Read the model definition and answer for the solid it produces. Units are mm, in the model's axes. Give positions to 0.01 mm unless a question says otherwise; leave off trailing zeros. Loops run counter-clockwise (first coordinate to the right, second up) from the corner with the lowest first, then second, coordinate; pieces in that order, holes last. Notation, with made-up numbers: (-23, 21.5) - (7, 21.5) arc R19 ccw to (7, 50.5) - close; hole circle Ø4 at (29.5, 15). An arc over 180 degrees is marked (long way). Use a Markdown table: item, result. Add a question column.
Item 1: A cutting plane is placed at B-B (y = 156.5). Determine the outline of the cut face in (x, z).
Item 2: A cutting plane is placed at A-A (x = -61). Determine the outline of the cut face in (y, z).
Item 3: Each of these flat-tipped pins is pushed along its axis until it touches: P1, Ø8, axis at x = -175, z = 13, coming from the -Y side; P2, Ø4, axis at y = -0.5, z = 42, coming from the -X side; P3, Ø10, axis at y = 182.5, z = 33.5, coming from the +X side. Where does it stop, or does it pass through?
Item 4: A cutting plane is placed at D-D (z = 12.5). Determine the outline of the cut face in (x, y), plus the area to 3 significant figures.
Item 5: Consider probe 1 along X at (y, z) = (-75.5, 23.5); probe 2 along Y at (x, z) = (-23.5, 40); probe 3 along X at (y, z) = (150, 26). Determine where each line is inside the solid, lowest interval first. Write a range as [from, to].
Item 6: A cutting plane is placed at C-C (z = 50). Determine the outline of the cut face in (x, y).
from build123d import *
from OCP.BRepAlgoAPI import BRepAlgoAPI_Cut
from OCP.TopTools import TopTools_ListOfShape

# Parameters (mm, degrees)
SKETCH1_W           = 500
SKETCH1_H           = 500
BOSS_EXTRUDE1_DEPTH = 60
FILLET3_R           = 50
FILLET4_R           = 50
FILLET6_START       = -234
FILLET6_DEPTH       = 502
FILLET6_2_DEPTH     = 492


with BuildPart() as part:
    # Sketch1 → Boss-Extrude1 (new body)
    with BuildSketch(Plane.XY):
        with Locations((11.616161616, 16.666666667)):
            Rectangle(SKETCH1_W, SKETCH1_H)
    extrude(amount=BOSS_EXTRUDE1_DEPTH)

    # Fillet3
    fillet3_edges = [part.edges().sort_by_distance(p)[0] for p in [
        (11.616161616, -233.333333333, 60),
        (261.616161616, 16.666666667, 60),
        (11.616161616, 266.666666667, 60),
        (-238.383838384, 16.666666667, 60),
    ]]
    fillet(fillet3_edges, radius=FILLET3_R)

    # Fillet4
    # the kernel refuses this fillet: 50 mm, written as the material it takes off along each edge
    with BuildSketch(Plane(origin=(-238.383838384, 341.666666667, 0), x_dir=(0, 0, 1), z_dir=(0, -1, 0)), Plane(origin=(336.616161616, 266.666666667, 0), x_dir=(0, 0, 1), z_dir=(-1, 0, 0))) as fillet4_piece_1:
        with BuildLine():
            CenterArc((50, -30), FILLET4_R, 143.130102354, 36.869897646)
            Line((0, -30), (-1, -30))
            Line((-1, -30), (-1, 0))
            Line((-1, 0), (0, 1))
            ThreePointArc((0, 1), (5, 1), (9.2, 0.6))
            Line((9.2, 0.6), (10, 0))
        make_face()
    extrude(amount=650, mode=Mode.SUBTRACT)
    with BuildSketch(Plane(origin=(-313.383838384, -233.333333333, 0), x_dir=(0, 1, 0), z_dir=(1, 0, 0)), Plane(origin=(261.616161616, -308.333333333, 0), x_dir=(-1, 0, 0), z_dir=(0, 1, 0))) as fillet4_piece_2:
        with BuildLine():
            CenterArc((30, 50), FILLET4_R, 233.130102354, 36.869897646)
            Line((0, 10), (-0.6, 9.2))
            ThreePointArc((-0.6, 9.2), (-1, 5), (-1, 0))
            Line((-1, 0), (0, -1))
            Line((0, -1), (30, -1))
            Line((30, -1), (30, 0))
        make_face()
    extrude(amount=650, mode=Mode.SUBTRACT)


with BuildPart() as fillet6_tool:
    # Fillet6: read off the stored shape, not the designer's step
    # Fillet6 outline → Fillet6 (new body)
    with BuildSketch(Plane(origin=(0, 0, 0), x_dir=(1, 0, 0), z_dir=(0, 1, 0)).offset(FILLET6_START)):
        with BuildLine():
            ThreePointArc((261.616161616, -10), (247.427549917, -2.565835097), (231.616161616, 0))
            ThreePointArc((231.616161616, 0), (253.976841391, -13.819660113), (251.616161616, -40))
            ThreePointArc((251.616161616, -40), (259.050326518, -25.811388301), (261.616161616, -10))
        make_face()
        with BuildLine():
            ThreePointArc((-228.383838384, -40), (-230.744518159, -13.819660113), (-208.383838384, 0))
            ThreePointArc((-208.383838384, 0), (-224.195226685, -2.565835097), (-238.383838384, -10))
            ThreePointArc((-238.383838384, -10), (-235.818003286, -25.811388301), (-228.383838384, -40))
        make_face()
    extrude(amount=FILLET6_DEPTH)


with BuildPart() as part_1:
    add(part.part)

    # Fillet6: cut by fillet6_tool, with a tolerance
    fillet6_stock = TopTools_ListOfShape()
    fillet6_stock.Append(part_1.part.wrapped)
    fillet6_tools = TopTools_ListOfShape()
    fillet6_tools.Append(fillet6_tool.part.wrapped)
    fillet6_cut = BRepAlgoAPI_Cut()
    fillet6_cut.SetArguments(fillet6_stock)
    fillet6_cut.SetTools(fillet6_tools)
    fillet6_cut.SetFuzzyValue(0.00001)
    fillet6_cut.Build()
    add(Compound.cast(fillet6_cut.Shape()).solids(), mode=Mode.REPLACE)


with BuildPart() as fillet6_2_tool:
    # Fillet6 2 outline → Fillet6 2 (new body)
    with BuildSketch(Plane.YZ.offset(FILLET6_START)):
        with BuildLine():
            ThreePointArc((-233.333333333, 10), (-219.144721634, 2.565835097), (-203.333333333, 0))
            ThreePointArc((-203.333333333, 0), (-225.694013108, 13.819660113), (-223.333333333, 40))
            ThreePointArc((-223.333333333, 40), (-230.767498236, 25.811388301), (-233.333333333, 10))
        make_face()
        with BuildLine():
            ThreePointArc((256.666666667, 40), (259.027346442, 13.819660113), (236.666666667, 0))
            ThreePointArc((236.666666667, 0), (252.478054612, 2.565834979), (266.666666667, 10))
            ThreePointArc((266.666666667, 10), (264.100831569, 25.811388301), (256.666666667, 40))
        make_face()
    extrude(amount=FILLET6_2_DEPTH)


with BuildPart() as part_2:
    add(part_1.part)

    # Fillet6 2: cut by fillet6_2_tool, with a tolerance
    fillet6_2_stock = TopTools_ListOfShape()
    fillet6_2_stock.Append(part_2.part.wrapped)
    fillet6_2_tools = TopTools_ListOfShape()
    fillet6_2_tools.Append(fillet6_2_tool.part.wrapped)
    fillet6_2_cut = BRepAlgoAPI_Cut()
    fillet6_2_cut.SetArguments(fillet6_2_stock)
    fillet6_2_cut.SetTools(fillet6_2_tools)
    fillet6_2_cut.SetFuzzyValue(0.00001)
    fillet6_2_cut.Build()
    add(Compound.cast(fillet6_2_cut.Shape()).solids(), mode=Mode.REPLACE)


solid = part_2.part
Geometry says:
| question | item | result |
|---|---|---|
| 1 | outline | (-228.38, 40) arc R25 ccw to (-208.38, 0) - (231.62, 0) arc R25 ccw to (251.62, 40) arc R50 ccw to (211.62, 60) - (-188.38, 60) arc R50 ccw to start |
| 2 | outline | (-223.33, 40) arc R25 ccw to (-203.33, 0) - (236.67, 0) arc R25 ccw to (256.67, 40) arc R50 ccw to (216.67, 60) - (-183.33, 60) arc R50 ccw to start |
| 3 | P1 | y = -227.02 |
| 3 | P2 | x = -228.38 |
| 3 | P3 | x = 256.37 |
| 4 | outline | (-230.03, -224.98) - (253.27, -224.98) - (253.27, 258.32) - (-230.03, 258.32) - close |
| 4 | area | 234,000 mm² |
| 5 | probe 1 | [-233.34, 256.57] |
| 5 | probe 2 | [-223.33, 256.67] |
| 5 | probe 3 | [-233.36, 256.6] |
| 6 | outline | (-218.38, -213.33) - (241.62, -213.33) - (241.62, 246.67) - (-218.38, 246.67) - close |
